Can you work these out from the model? Positions are in its coordinate system, mm. Face numbers are marked on the shaded views. A direction names the side the tool comes from. Coordinates: 2 decimals unless noted, no trailing zeros. Order: outer loops, then holes, each group sorted by start corner. A loop starts at its lowest first (then second) coordinate and runs counter-clockwise, first axis right, second up. Notation, with made-up numbers: (3, 79.25) -> (8, 79.25) arc R21 cw to (8, 100.25) -> close; hole circle Ø9 at (74.25, 72). An arc over 180 degrees is marked (long way). Return JSON: item names as keys, results as strings. Group by question number.
1) If I drill on probe 1 along X at (y, z) = (18, 1.5); probe 2 along X at (y, z) = (14, -31); probe 3 along Y at (x, z) = (13, -10), over which ranges is the centre line in solid material (lowest first)? Write a range as from..to.
2) For the marked faces 1, 2 and 3, which set-ups out of +Z, -Z, +X, -X, +Y, -Y let a thin tool reach every point of the face, with its end or its side?
3) Thinking about a two-plate mould opening in Z: for the marked faces 4, 5 and 6, which applies, +Z half, -Z half, draft (parallel to the pull), parting line (faces both ways), or undercut?
4) If we section it at A-A, the plane y = 10: Please give me the cut outline in (x, z), then the cut area to 3 significant figures.
5) If we section it at C-C, the plane z = 10: Please give me the cut outline in (x, y), then the cut area to 3 significant figures.
6) If we section it at B-B, the plane z = 0: Please give me the cut outline in (x, y), then the cut area to 3 significant figures.
7) For pin 1 (8 mm diameter, centred on x = 86, z = 1.5, fed in from -Y); pin 2 (6 mm diameter, centred on x = 25, z = 27, fed in from -Y); pin 3 (10 mm diameter, centred on y = 12.5, z = 28, fed in from +X), each with a flat end and sliding along its axis, tell me the tip position at first contact or that it passes through.
from build123d import *

# Parameters (mm, degrees)
SKETCH_2_R          = 5
CUT_EXTRUDE_1_DEPTH = 20
SKETCH_3_R          = 5
CUT_EXTRUDE_2_DEPTH = 112.579568022


with BuildPart() as part:
    # Эскиз1 → Повернуть1 (revolve)
    with BuildSketch(Plane.XY, mode=Mode.PRIVATE) as revolve_1_sk:
        Polygon((0, 0), (100, 0), (100, 15), (40, 15), (40, 35), (10, 35), (10, 20), (0, 20), align=None)
    revolve(revolve_1_sk.sketch.rotate(Axis((0, 0, 0), (1, 0, 0)), 90), axis=Axis((0, 0, 0), (1, 0, 0)))

    # Эскиз2 → Вырез-Вытянуть1 (cut)
    with BuildSketch(Plane(origin=(0, 0, 0), x_dir=(0, 0, -1), z_dir=(1, 0, 0))):
        with Locations((10, 10)):
            Circle(SKETCH_2_R)
    extrude(amount=CUT_EXTRUDE_1_DEPTH, mode=Mode.SUBTRACT)

    # Эскиз3 → Вырез-Вытянуть2 (cut, through all)
    with BuildSketch(Plane(origin=(0, 0, 0), x_dir=(0, 0, -1), z_dir=(1, 0, 0))):
        with Locations(Location((-10, 10, 0), (0, 0, 225))):
            Circle(SKETCH_3_R)
    extrude(amount=CUT_EXTRUDE_2_DEPTH, mode=Mode.SUBTRACT)


solid = part.part
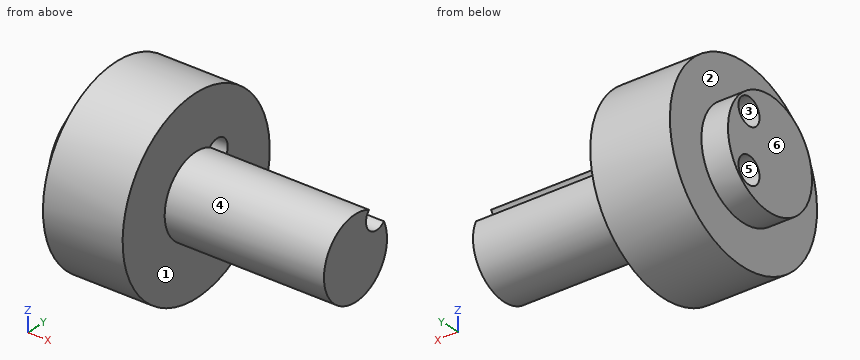
Result sheet:
{
 "1": {"probe 1": "x = 0..40", "probe 2": "x = 10..40", "probe 3": "y = -33.54..5, 15..33.54"},
 "2": {"face 1": "+X", "face 2": "-X", "face 3": "+X, -X"},
 "3": {"face 4": "parting line", "face 5": "undercut", "face 6": "draft"},
 "4": {"outline": "(0, -17.32) -> (10, -17.32) -> (10, -33.54) -> (40, -33.54) -> (40, -11.18) -> (100, -11.18) -> (100, 5) -> (0, 5) -> (0, -5) -> (20, -5) -> (20, -15) -> (0, -15) -> close; (0, 15) -> (40, 15) -> (40, 33.54) -> (10, 33.54) -> (10, 17.32) -> (0, 17.32) -> close", "area": "2,730 mm2"},
 "5": {"outline": "(0, -17.32) -> (10, -17.32) -> (10, -33.54) -> (40, -33.54) -> (40, -11.18) -> (100, -11.18) -> (100, 5) -> (0, 5) -> close; (0, 15) -> (40, 15) -> (40, 33.54) -> (10, 33.54) -> (10, 17.32) -> (0, 17.32) -> close", "area": "2,930 mm2"},
 "6": {"outline": "(0, -20) -> (10, -20) -> (10, -35) -> (40, -35) -> (40, -15) -> (100, -15) -> (100, 15) -> (40, 15) -> (40, 35) -> (10, 35) -> (10, 20) -> (0, 20) -> close", "area": "4,300 mm2"},
 "7": {"pin 1": "stops at y = -15", "pin 2": "stops at y = -25.48", "pin 3": "stops at x = 40"}
}
